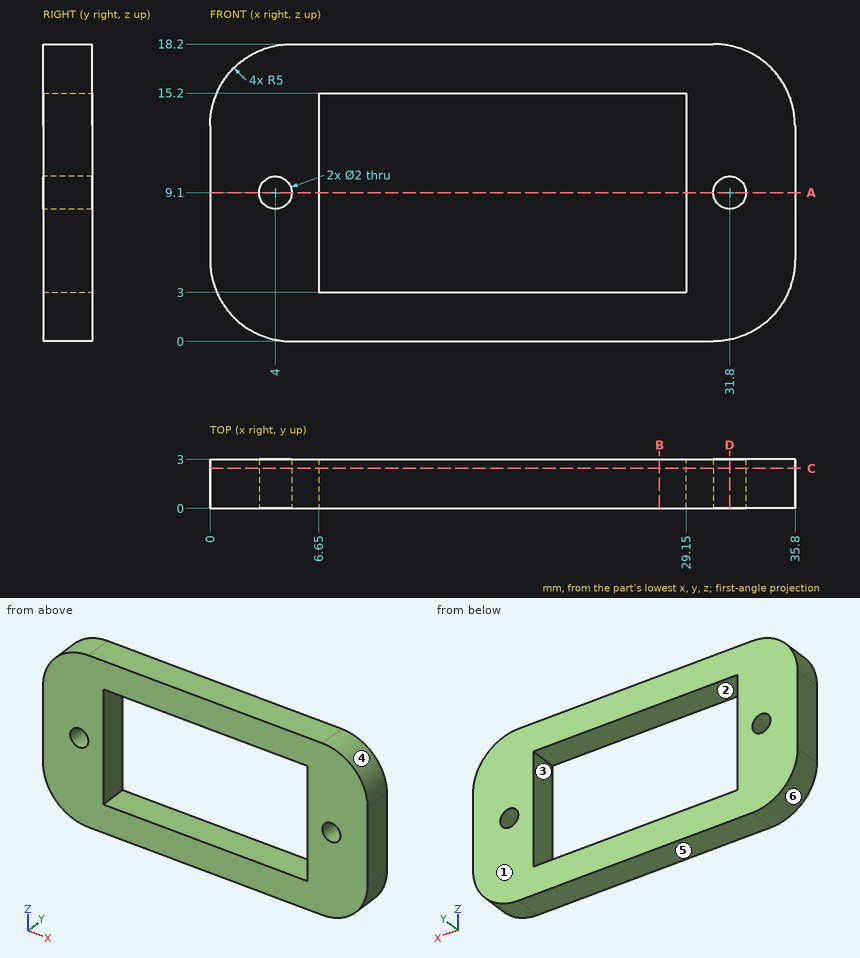
Input: dimensioned drawing with shaded views. Units: mm. Origin: part minimum x, y, z. A direction names the side the tool comes from. Give positions to 0.01 mm unless a question says otherwise; leave off trailing zeros. Loops run counter-clockwise (first coordinate to the right, second up) from the corner with the lowest first, then second, coordinate; pieces in that order, holes last. Notation, with made-up numbers: (-28, 40.25) - (-16, 40.25) arc R26 cw to (-16, 57.25) - close; hole circle Ø8 at (3.25, 82). An arc over 180 degrees is marked (long way). Answer as CSV lines item,"result". Start each with the question number.
(1) Ray query, line 1 along X through (y, z) = (1.1, 7.25); line 2 along Z through (x, y) = (16.5, 0.9); line 3 along X through (y, z) = (0.7, 8.75). Return the intervals inside material, ascending. Write a range as [from, to].
(2) Mould query, pull axis X, two halves, no side actions, for the marked faces 3, 4, 5 and 6. Classes: +X half, -X half, draft (parallel to the pull), parting line (faces both ways), or undercut.
(3) Section query D-D (x = 31.8). Output: boundary loops of the cut face in (y, z), and give its area (3 significant figures).
(4) Reachability of the marked faces 1 and 2 from +Z, -Z, +X, -X, +Y, -Y: full face, straight path, thin tool, end or side. Return the list, or none.
(5) Section query C-C (y = 2.45). Output: boundary loops of the cut face in (x, z), and give its area (3 significant figures).
(6) Section query B-B (x = 27.5). Output: boundary loops of the cut face in (y, z).
(7) Section query A-A (z = 9.1). Output: boundary loops of the cut face in (x, y), and give its area (3 significant figures).
Worked answers:
1,line 1,"x = [0, 6.65], [29.15, 35.8]"
1,line 2,"z = [0, 3], [15.2, 18.2]"
1,line 3,"x = [0, 3.06], [4.94, 6.65], [29.15, 30.86], [32.74, 35.8]"
2,face 3,"undercut"
2,face 4,"+X half"
2,face 5,"draft"
2,face 6,"-X half"
3,outline,"(0, 0.1) - (3, 0.1) - (3, 8.1) - (0, 8.1) - close; (0, 10.1) - (3, 10.1) - (3, 18.1) - (0, 18.1) - close"
3,area,"48.0 mm^2"
4,face 1,"+Z, -Z, +X, -X, +Y"
4,face 2,"+Y, -Y"
5,outline,"(0, 5) arc R5 ccw to (5, 0) - (30.8, 0) arc R5 ccw to (35.8, 5) - (35.8, 13.2) arc R5 ccw to (30.8, 18.2) - (5, 18.2) arc R5 ccw to (0, 13.2) - close; hole circle Ø2 at (4, 9.1); hole (6.65, 3) - (29.15, 3) - (29.15, 15.2) - (6.65, 15.2) - close; hole circle Ø2 at (31.8, 9.1)"
5,area,"349 mm^2"
6,outline,"(0, 0) - (3, 0) - (3, 3) - (0, 3) - close; (0, 15.2) - (3, 15.2) - (3, 18.2) - (0, 18.2) - close"
7,outline,"(0, 0) - (3, 0) - (3, 3) - (0, 3) - close; (5, 0) - (6.65, 0) - (6.65, 3) - (5, 3) - close; (29.15, 0) - (30.8, 0) - (30.8, 3) - (29.15, 3) - close; (32.8, 0) - (35.8, 0) - (35.8, 3) - (32.8, 3) - close"
7,area,"27.9 mm^2"
